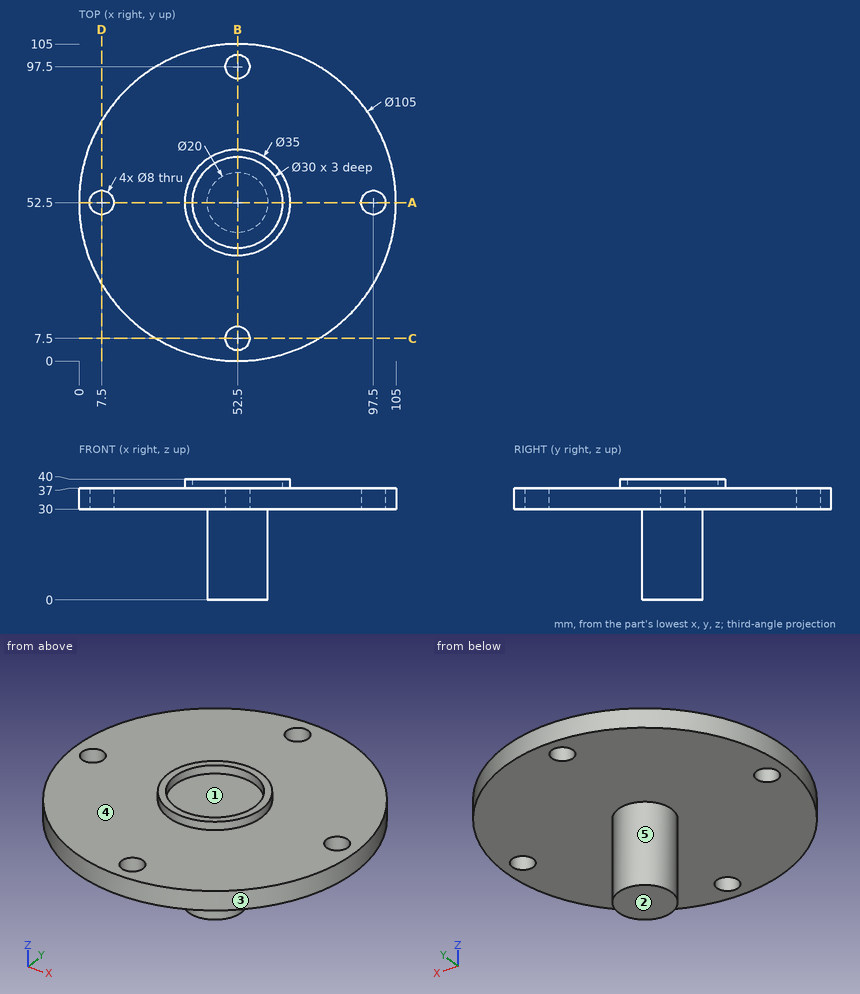
Part print with two shaded views. Sizes in mm from the minimum x, y, z corner. A direction names the side the tool comes from. Round coordinates to 2 decimals unless told otherwise and drop trailing zeros. Order: outer loops, then holes, each group sorted by start corner. A loop starts at its lowest first (then second) coordinate and runs counter-clockwise, first axis right, second up.
(1) Drill centre lines: line 1 (Y direction, x = 52, z = 32); line 2 (Y direction, x = 52.5, z = 39.35). Where is each one in solid material? Low to high.
(2) Pull direction Y, two halves, no side cores. Call the marked faces 1, 2 and 3: released by +Y, released by -Y, zero draft, split by the parting line, or undercut.
(3) 3-axis set-ups, long thin cutter, end or side, ignore diameter. For the marked faces 4 and 5: which of +Z, -Z, +X, -X, +Y, -Y reach the whole face in a straight line?
(4) Band-saw the part on C-C (y = 7.5). List the corners of the cut face in (x, z).
(5) Band-saw the part on A-A (y = 52.5). List the corners of the cut face in (x, z).
(6) Pin check, flat tips, straight feed: pin 1 (9 mm diameter, centred on x = 51, y = 54.5, fed in from +Z); pin 2 (5 mm diameter, centred on x = 41.5, z = 7.5, fed in from +Y); pin 3 (5 mm diameter, centred on x = 88.5, y = 17.5, fed in from -Z). Stop position of each tip, or through.
Verdict:
1. line 1: y = 0 to 3.53, 11.47 to 93.53, 101.47 to 105
1. line 2: y = 35 to 37.5, 67.5 to 70
2. face 1: undercut
2. face 2: zero draft
2. face 3: split by the parting line
3. face 4: +Z
3. face 5: -Z
4. outline: (25.46, 30) - (48.5, 30) - (48.5, 37) - (25.46, 37) - close; (56.5, 30) - (79.54, 30) - (79.54, 37) - (56.5, 37) - close
5. outline: (0, 30) - (3.5, 30) - (3.5, 37) - (0, 37) - close; (11.5, 30) - (42.5, 30) - (42.5, 0) - (62.5, 0) - (62.5, 30) - (93.5, 30) - (93.5, 37) - (70, 37) - (70, 40) - (67.5, 40) - (67.5, 37) - (37.5, 37) - (37.5, 40) - (35, 40) - (35, 37) - (11.5, 37) - close; (101.5, 30) - (105, 30) - (105, 37) - (101.5, 37) - close
6. pin 1: stops at z = 37
6. pin 2: stops at y = 57.77
6. pin 3: stops at z = 30
